Read the model definition and answer for the solid it produces. Units are mm, in the model's axes. A direction names the side the tool comes from. Round coordinates to 2 decimals unless told otherwise and drop trailing zeros. Order: outer loops, then holes, each group sorted by start corner. A loop starts at its lowest first (then second) coordinate and runs counter-clockwise, first axis right, second up. Notation, with made-up numbers: (26, 86.25) -> (39, 86.25) arc R17 cw to (39, 110.25) -> close; hole circle Ø3 at (55, 10). An arc over 180 degrees is marked (long way). One line per item, written item: value. Start each with the question number.
1. Consider line 1 (Y direction, x = 0, z = 2); line 2 (X direction, y = 0, z = 1.35); line 3 (Z direction, x = -20.5, y = 5). Determine where each line is inside the solid, lowest interval first.
2. Section A-A (x = 0) is taken. Give the vertices of the cut face in (y, z), then the cut area to 3 significant figures.
3. Section C-C (y = -48) is taken. Give the vertices of the cut face in (x, z).
4. Section B-B (y = 0) is taken. Give the vertices of the cut face in (x, z).
5. Section D-D (z = 27) is taken. Give the vertices of the cut face in (x, y).
6. Flat-ended cylindrical pins translate along their axes: pin 1 Ø18 at (x, y) = (0, 0) entering from +Z; pin 2 Ø10 at (y, z) = (-15.5, 8.5) entering from -X; pin 3 Ø1 at (x, z) = (6, 27) entering from -Y; pin 4 Ø12 at (x, z) = (-15, 18) entering from +Y. Find the tip coordinate at first contact, or state that the pin passes through.
7. For faces 1 (the face through (-2.17, -9.76, 1.48)), 2 (the face through (5, 13, 3)), 3 (the face through (24, -1, 1)), determine the directions among +Z, -Z, +X, -X, +Y, -Y from which every point of the face is accessible in a straight line to the end or side of a thin tool.
8. The mould has two halves that part along X. Classify faces 4 (the face through (-23.4, 52.43, 1.48)), 5 (the face through (0, 53, 1)), 6 (the face through (0, 44, 1)), 7 (the face through (2, 4, 30)): released by +X, released by -X, zero draft, split by the parting line, or undercut.
from build123d import *

# Parameters (mm, degrees)
F0_R     = 1
F0_R_2   = 10
F1_DEPTH = 3
F4_R     = 4
F5_DEPTH = 33.001


with BuildPart() as f1:
    # F0 (on Top) → F1 (new body)
    with BuildSketch(Plane.XY):
        with BuildLine():
            Line((22, 53), (-22, 53))
            ThreePointArc((-22, 53), (-23.414214, 52.414214), (-24, 51))
            Line((-24, 51), (-24, -51))
            ThreePointArc((-24, -51), (-23.414214, -52.414214), (-22, -53))
            Line((-22, -53), (22, -53))
            ThreePointArc((22, -53), (23.414214, -52.414214), (24, -51))
            Line((24, -51), (24, 51))
            ThreePointArc((24, 51), (23.414214, 52.414214), (22, 53))
        make_face()
        with Locations((0, -48)):
            Circle(F0_R, mode=Mode.SUBTRACT)
        Circle(F0_R_2, mode=Mode.SUBTRACT)
        with Locations((0, 43)):
            Circle(F0_R, mode=Mode.SUBTRACT)
    extrude(amount=F1_DEPTH)

    # F2 (on Right) → F3 (revolve)
    with BuildSketch(Plane.YZ):
        Polygon((8, 30), (10, 3), (13.008219, 3), (10.785997, 33), (0, 33), (0, 30), align=None)
    revolve(axis=Axis((0, 0, 4.326884), (0, 0, 1)))

    # F4 (on face) → F5 (cut, through all)
    with BuildSketch(Plane.XY.offset(33)):
        Circle(F4_R)
    extrude(amount=-F5_DEPTH, mode=Mode.SUBTRACT)


solid = f1.part
Answer:
1. line 1: -53 to -49, -47 to -10, 10 to 42, 44 to 53
1. line 2: -24 to -10, 10 to 24
1. line 3: 0 to 3
2. outline: (-53, 0) -> (-49, 0) -> (-49, 3) -> (-53, 3) -> close; (-47, 0) -> (-10, 0) -> (-10, 3) -> (-8, 30) -> (-4, 30) -> (-4, 33) -> (-10.79, 33) -> (-13.01, 3) -> (-47, 3) -> close; (4, 30) -> (8, 30) -> (10, 3) -> (10, 0) -> (42, 0) -> (42, 3) -> (13.01, 3) -> (10.79, 33) -> (4, 33) -> close; (44, 0) -> (53, 0) -> (53, 3) -> (44, 3) -> close
2. area: 450 mm^2
3. outline: (-24, 0) -> (-1, 0) -> (-1, 3) -> (-24, 3) -> close; (1, 0) -> (24, 0) -> (24, 3) -> (1, 3) -> close
4. outline: (-24, 0) -> (-10, 0) -> (-10, 3) -> (-8, 30) -> (-4, 30) -> (-4, 33) -> (-10.79, 33) -> (-13.01, 3) -> (-24, 3) -> close; (4, 30) -> (8, 30) -> (10, 3) -> (10, 0) -> (24, 0) -> (24, 3) -> (13.01, 3) -> (10.79, 33) -> (4, 33) -> close
5. outline: circle Ø22.46 at (0, 0); hole circle Ø16.44 at (0, 0)
6. pin 1: z = 33
6. pin 2: x = -7
6. pin 3: y = -9.79
6. pin 4: y = 7.81
7. face 1: -Z
7. face 2: +Z
7. face 3: +Z, -Z, +X, +Y, -Y
8. face 4: released by -X
8. face 5: zero draft
8. face 6: undercut
8. face 7: undercut
